Autodesk Inventor part; units mm, degrees
ref_plane "Work Plane1" through (30.1625, 0, 0) normal (0, 0, -1) x (1, 0, 0)
ref_plane "YZ Plane" through (0, 0, 0) normal (1, 0, 0) x (0, 1, 0)
ref_plane "XZ Plane" through (0, 0, 0) normal (0, 1, 0) x (-1, 0, 0)
sketch "Sketch1" plane through (0, 0, 0) normal (0, 0, 1) x (1, 0, 0)
  line L0 (-3, 0) -> (8, 0)
  line L1 (8, 0) -> (8, 2.5)
  line L2 (8, 2.5) -> (1.6, 2.5)
  line L3 (1.6, 2.5) -> (1.1091, 2.2547)
  line L4 (1.1091, 2.2547) -> (0, 2.2547)
  line L5 (0, 2.2547) -> (0, 4.75)
  line L6 (-5.2, 0) -> (10.2, 0)
  line L7 (0, -0.95) -> (0, 5.7)
  line L8 (-3, 0) -> (-3, 4.4875)
  line L9 (0, 4.75) -> (-3, 4.4875)
  line L10 (1.6, 2.5) -> (0, 2.5) construction
  dimension "d0" = 8
  dimension "d1" = 6.4
  dimension "d2" = 0.4909
  dimension "d3" = 3
  dimension "d4" = 5
  dimension "d5" = 4.5095
  dimension "d9" = 9.5
  dimension "d10" = 5
revolve "Body" add sketch "Sketch1" angle 360 about axis through (-3, 0, 0) along (1, 0, 0)
sketch "Sketch2" plane through (-3, 0, 0) normal (-1, 0, 0) x (0, 0, 1)
  circle A0 centre (0, 0) radius 4.75
  line L0 (0, 0) -> (0, 4.4875)
  line L1 (-4.75, 0.6) -> (4.75, 0.6)
  line L2 (4.75, 0.6) -> (4.75, -0.6)
  line L3 (4.75, -0.6) -> (-4.75, -0.6)
  line L4 (-4.75, -0.6) -> (-4.75, 0.6)
  line L5 (-4.75, 0) -> (4.75, 0) construction
  line L6 (0, 0.6) -> (0, -0.6) construction
  dimension "d11" = 1.2
  dimension "d12" = 9.5
fillet "Fillet1" radius 1.5 1 edges at (-3, -4.4875, 0)
extrude "Slot" cut sketch "Sketch2" against normal blind 1.2 contours A0 L3 L1 | L2 L3 A0 | A0 L1 L2 | A0 L4 L1 | L3 L4 A0
thread "Thread"
ref_plane "Work Plane1" through (30.1625, 0, 0) normal (0, 0, -1) x (1, 0, 0)
fillet "Fillet5" radius 0.2 1 edges at (0, -2.2547, 0)
equation "\"d11\" = SBR"
equation "\"d12\" = KOD"
equation "\"d14\" = RR"
equation "\"d19\" = STI"
equation "\"d15\" = GEL"
equation "\"d41\" = R"
equation "\"d0\" = NLG"
equation "\"d1\" = GEL"
equation "\"d3\" = KOH"
equation "\"d4\" = GD"
equation "\"d5\" = BDM"
equation "\"d9\" = KOD"
equation "\"d10\" = KEWI"
equation "\"GD\" = NND"
equation "\"NLG\" = 8"
equation "\"GEL\" = 6.4"
equation "\"KOD\" = 9.5"
equation "\"KOH\" = 3"
equation "\"GAL\" = 0.61345 * PTC"
equation "\"R\" = 0.2"
equation "\"BDM\" = 4.5095"
equation "\"GUL\" = 0.61345 * PTC"
equation "\"RR\" = 1.5"
equation "\"SBR\" = 1.2"
equation "\"STI\" = 1.2"
equation "\"KEWI\" = 5deg"
equation "\"PTC\" = 0.8"
equation "\"THREADDIA\" = 5"
equation "\"TOA\" = 30deg"
equation "\"NND\" = 5"
equation "\"GD1\" = THREADDIA - 1.2269 * PTC"
properties part number "ISO 1580 - M5 x 8" material "Steel, Mild"
CAD build for the part. Positions are in the model's coordinates, mm. A direction names the side the tool comes from. Round coordinates to 2 decimals unless told otherwise and drop trailing zeros. Order: outer loops, then holes, each group sorted by start corner. A loop starts at its lowest first (then second) coordinate and runs counter-clockwise, first axis right, second up.
Item 1: Saw through at A-A on z = 0. Write the cut outline in (x, y).
Item 2: Pin check, flat tips, straight feed: pin 1 (4 mm diameter, centred on x = 1, y = 2, fed in from -Z); pin 2 (1 mm diameter, centred on x = -2.5, z = 1, fed in from -Y); pin 3 (0.6 mm diameter, centred on x = -2.5, z = 2, fed in from +Y). Stop position of each tip, or through.
Item 3: Probe line 1 along X through (y, z) = (0.5, 0.25); line 2 along X through (y, z) = (0.75, 2.75); line 3 along Y through (x, z) = (-1.75, -4). List the from-to ranges inside material, lowest first.
Item 4: Saw through at B-B on y = 0. Write the cut outline in (x, z).
Item 5: Mould opens along X. For faces 1 (the face through (8, 0, 0)), 2 (the face through (0.65, -1.79, 1.37)), 3 (the face through (-2, 0.6, 0)) say: pulls with the +X half, pulls with the -X half, needs draft (parallel to the pull), parting line crosses it, or undercut.
Item 6: Saw through at D-D on x = 4.25. Write the cut outline in (y, z).
Item 7: Saw through at C-C on x = -2. Write the cut outline in (y, z).
Item 8: Tool access for faces 4 (the face through (-3, -2, 0)), 5 (the face through (-2, -0.6, 0)), 6 (the face through (4.76, -0.54, 2.44)): list every direction of +Z, -Z, +X, -X, +Y, -Y with a clear straight run to the whole face (end or side of a thin tool).
Reported:
1. outline: (-3, -3.11) arc R1.5 ccw to (-1.63, -4.61) - (0, -4.75) - (0, -2.45) arc R0.2 cw to (0.2, -2.25) - (1.11, -2.25) - (1.6, -2.5) - (8, -2.5) - (8, 2.5) - (1.6, 2.5) - (1.11, 2.25) - (0.2, 2.25) arc R0.2 cw to (0, 2.45) - (0, 4.75) - (-1.63, 4.61) arc R1.5 ccw to (-3, 3.11) - (-3, 0.6) - (-1.8, 0.6) - (-1.8, -0.6) - (-3, -0.6) - close
2. pin 1: stops at z = -4.74
2. pin 2: stops at y = -4.44
2. pin 3: stops at y = 4.01
3. line 1: x = -1.8 to 8
3. line 2: x = -3 to 0
3. line 3: y = -2.26 to 2.26
4. outline: (-1.8, -4.58) arc R1.5 ccw to (-1.63, -4.61) - (0, -4.75) - (0, -2.45) arc R0.2 cw to (0.2, -2.25) - (1.11, -2.25) - (1.6, -2.5) - (8, -2.5) - (8, 2.5) - (1.6, 2.5) - (1.11, 2.25) - (0.2, 2.25) arc R0.2 cw to (0, 2.45) - (0, 4.75) - (-1.63, 4.61) arc R1.5 ccw to (-1.8, 4.58) - close
5. face 1: pulls with the +X half
5. face 2: undercut
5. face 3: needs draft
6. outline: circle Ø5 at (0, 0)
7. outline: (-0.6, -4.49) - (-0.6, 4.49) arc R4.53 ccw to start; (0.6, -4.49) arc R4.53 ccw to (0.6, 4.49) - close
8. face 4: +Z, -Z, -X, +Y, -Y
8. face 5: +Z, -Z, -X
8. face 6: +X
